Design review of the part built by this model. Coordinates are the model's own, in mm. A direction names the side the tool comes from. Coordinates: 2 decimals unless noted, no trailing zeros. Write each loop counter-clockwise with the first axis right and the second up, starting at its lowest first coordinate (ties: lowest second). Pieces come first, ordered by that corner, then holes.
Q1. Take a section at A-A (z = 5). Give the boundary of the cut face in (x, y).
Q2. Mouldability with a two-part tool opening along X and no side actions: class faces 4 (the flat face through (0, 0, 11)), 5 (the cylindrical face through (-2.43, 2.23, 1.97)), 6 (the cylindrical face through (-1.604, 0.071, 7.549)), 7 (the cylindrical face through (1.1, -1.9, 4)) as pulls with the +X half, pulls with the -X half, needs draft (parallel to the pull), parting line crosses it, or undercut.
Q3. Machinability: for faces 1 (the conical face through (-2.356, 1.378, 8.229)), 2 (the flat face through (2.4, 0.4, 8.4)), 3 (the cylindrical face through (-1.725, 1.013, 7.549)), which of the approach directions +Z, -Z, +X, -X, +Y, -Y give a long, thin tool a straight path to every point of the face, cutting with its end or side? Answer none if there is none.
Q4. Take a section at B-B (x = 0). Give the boundary of the cut face in (y, z), and give its area (3 significant figures).
Q5. Take a section at C-C (y = 0.25). Give the boundary of the cut face in (x, z), and give its area (3 significant figures).
Q6. Insertion check: pin 1 (1.5 mm diameter, centred on y = 1.5, z = 6.5, fed in from +X); pin 2 (0.9 mm diameter, centred on x = -2.5, z = 8, fed in from +Y); pin 3 (0.6 mm diameter, centred on x = 2.5, z = 9.5, fed in from -Y); pin 4 (2 mm diameter, centred on y = 0.5, z = 2.5, fed in from +X). Each pin has a flat end and moves straight along its axis. Give the tip position at first contact, or say it passes through.
Q7. For probe 1 along Y at (x, z) = (2.25, 10.75); probe 2 along Y at (x, z) = (0.5, 9); probe 3 along Y at (x, z) = (0.5, 7.75), list the stretches that pass through material, from the lowest coordinate up.
Q8. Take a section at D-D (z = 3). Give the boundary of the cut face in (x, y).
```python
from build123d import *

# Parameters (mm, degrees)
SKETCH004_R          = 2.5
PAD001_DEPTH         = 11
POCKET003_DEPTH      = 5
POCKET003_DEPTH_BACK = 5
POLARPATTERN_COUNT   = 3
SKETCH007_R          = 2
POCKET004_DEPTH      = 7
SKETCH008_R          = 1.605124
PAD002_DEPTH         = 7


with BuildPart() as part:
    # Sketch004 → Pad001 (new body)
    with BuildSketch(Plane.XY):
        Circle(SKETCH004_R)
    extrude(amount=PAD001_DEPTH)

    # Sketch005 → Revolution (revolve)
    with BuildSketch(Plane.XZ):
        Polygon((2.5, 11), (3.1, 10.4), (3.1, 8.6), (2.5, 8), align=None)
        Polygon((2.5, 1.5), (2.3, 1.5), (2.3, 4), (3.3, 4), (3.3, 0), (2.5, 0), align=None)
    revolve(axis=Axis((0, 0, 0), (0, 0, 1)))

    # Sketch006 → Pocket003 (cut, two sides)
    with BuildSketch(Plane.YZ) as pocket003_sk:
        with BuildLine():
            ThreePointArc((-0.4, 4.4), (0, 4), (0.4, 4.4))
            Line((0.4, 4.4), (0.4, 14.4))
            ThreePointArc((0.4, 14.4), (0, 14.8), (-0.4, 14.4))
            Line((-0.4, 4.4), (-0.4, 14.4))
        make_face()
    pocket003 = extrude(amount=-POCKET003_DEPTH, mode=Mode.SUBTRACT) + extrude(pocket003_sk.sketch, amount=POCKET003_DEPTH_BACK, mode=Mode.SUBTRACT)

    # PolarPattern: Pocket003 ×3 about axis
    polarpattern_axis = Axis((0, 0, 0), (0, 0, 1))
    for i in range(1, POLARPATTERN_COUNT):
        add(pocket003.rotate(polarpattern_axis, i * 360 / POLARPATTERN_COUNT), mode=Mode.SUBTRACT)

    # Sketch007 (on Face49 of PolarPattern) → Pocket004 (cut)
    with BuildSketch(Plane.XY.offset(11)):
        Circle(SKETCH007_R)
    extrude(amount=-POCKET004_DEPTH, mode=Mode.SUBTRACT)

    # Sketch008 (on Face46 of Pocket004) → Pad002 (join)
    with BuildSketch(Plane.XY.offset(11)):
        Circle(SKETCH008_R)
    extrude(amount=-PAD002_DEPTH)


solid = part.part
```
Response:
1. outline: (-2.47, -0.4) arc R2.5 ccw to (-1.58, -1.94) - (-1.33, -1.5) arc R2 cw to (-1.96, -0.4) - close; (-2.47, 0.4) - (-1.96, 0.4) arc R2 cw to (-1.33, 1.5) - (-1.58, 1.94) arc R2.5 ccw to start; circle Ø3.21 at (0, 0); (-0.89, -2.34) arc R2.5 ccw to (0.89, -2.34) - (0.63, -1.9) arc R2 cw to (-0.63, -1.9) - close; (-0.89, 2.34) - (-0.63, 1.9) arc R2 cw to (0.63, 1.9) - (0.89, 2.34) arc R2.5 ccw to start; (1.33, -1.5) - (1.58, -1.94) arc R2.5 ccw to (2.47, -0.4) - (1.96, -0.4) arc R2 cw to start; (1.33, 1.5) arc R2 cw to (1.96, 0.4) - (2.47, 0.4) arc R2.5 ccw to (1.58, 1.94) - close
2. face 4: needs draft
2. face 5: parting line crosses it
2. face 6: undercut
2. face 7: undercut
3. face 1: -X, +Y
3. face 2: +Z, +X
3. face 3: +Z
4. outline: (-3.3, 0) - (3.3, 0) - (3.3, 4) - (2.5, 4) - (2.5, 8) - (3.1, 8.6) - (3.1, 10.4) - (2.5, 11) - (2, 11) - (2, 4) - (1.61, 4) - (1.61, 11) - (-1.61, 11) - (-1.61, 4) - (-2, 4) - (-2, 11) - (-2.5, 11) - (-3.1, 10.4) - (-3.1, 8.6) - (-2.5, 8) - (-2.5, 4) - (-3.3, 4) - close
4. area: 58.8 mm2
5. outline: (-3.29, 0) - (3.29, 0) - (3.29, 4) - (2.49, 4) - (2.49, 4.09) - (1.98, 4.09) - (1.98, 4) - (1.59, 4) - (1.59, 11) - (-1.59, 11) - (-1.59, 4) - (-1.98, 4) - (-1.98, 4.09) - (-2.49, 4.09) - (-2.49, 4) - (-3.29, 4) - close
5. area: 48.6 mm2
6. pin 1: stops at x = 2.38
6. pin 2: stops at y = 1.79
6. pin 3: stops at y = -2.18
6. pin 4: stops at x = 3.3
7. probe 1: y = -1.58 to -0.4, 0.4 to 1.58
7. probe 2: y = -3.06 to -1.94, -1.53 to 1.53, 1.94 to 3.06
7. probe 3: y = -2.45 to -1.94, -1.53 to 1.53, 1.94 to 2.45
8. outline: circle Ø6.6 at (0, 0)
